Autodesk Inventor part; units mm, degrees
ref_plane "YZ Plane" through (0, 0, 0) normal (1, 0, 0) x (0, 1, 0)
ref_plane "XZ Plane" through (0, 0, 0) normal (0, 1, 0) x (-1, 0, 0)
ref_plane "XY Plane" through (0, 0, 0) normal (0, 0, 1) x (1, 0, 0)
sketch "Skizze2" plane through (0, 0, 0) normal (1, 0, 0) x (0, 1, 0)
  line L0 (1.25, 6) -> (-1.25, 6)
  line L1 (-1.25, 6) -> (-1.25, 0.25)
  line L2 (-1.25, 0.25) -> (-0.95, 0.25)
  line L3 (-0.95, 0.25) -> (-0.95, -0.25)
  line L4 (-0.95, -0.25) -> (-1.25, -0.25)
  line L5 (-1.25, -0.25) -> (-1.25, -6)
  line L6 (-1.25, -6) -> (1.25, -6)
  line L7 (1.25, -6) -> (1.25, -0.25)
  line L8 (1.25, -0.25) -> (0.95, -0.25)
  line L9 (0.95, -0.25) -> (0.95, 0.25)
  line L10 (0.95, 0.25) -> (1.25, 0.25)
  line L11 (1.25, 0.25) -> (1.25, 6)
  line L12 (0.25, 6) -> (0.25, -6) construction
  line L13 (-0.25, -6) -> (-0.25, 6) construction
  point P0 (0, 0)
  point P1 (0.95, 0)
  dimension "d0" = 0.5
  dimension "d1" = 1
  dimension "d2" = 1
  dimension "d3" = 0.5
  dimension "d4" = 0.25
  dimension "d5" = 0.3
  dimension "d6" = 0.3
  dimension "d7" = 6
  dimension "d8" = 6
extrude "Extrusion1" add sketch "Skizze2" along normal mid plane 12
sketch "Skizze3" plane through (-6, -1.25, -6) normal (0, 0, -1) x (-1, 0, 0)
  line L0 (-11, 1.5) -> (-1, 1.5)
  line L1 (-1, 1.5) -> (-1, 1)
  line L2 (-1, 1) -> (-11, 1)
  line L3 (-11, 1) -> (-11, 1.5)
  line L4 (0, 2.5) -> (-12, 2.5)
  line L5 (0, 2.5) -> (0, 0)
  point P0 (-6, 1.25)
  point P1 (-6, 1.5)
  point P2 (-6, 2.5)
  point P3 (-1, 1.25)
  point P4 (0, 1.25)
  dimension "d11" = 10
  dimension "d12" = 0.5
extrude "Extrusion2" cut sketch "Skizze3" against normal blind 12
sketch "Skizze4" plane through (-5, -0.25, -6) normal (0, 1, 0) x (1, 0, 0)
  line L0 (-1, -12) -> (11, -12)
  line L1 (-1, 0) -> (11, 0)
  line L2 (4.3, 0) -> (5.7, 0)
  line L3 (5.7, 0) -> (5.7, -12)
  line L4 (5.7, -12) -> (4.3, -12)
  line L5 (4.3, -12) -> (4.3, 0)
  line L6 (3.3, -12) -> (1.9, -12)
  line L7 (1.9, -12) -> (1.9, 0)
  line L8 (1.9, 0) -> (3.3, 0)
  line L9 (3.3, 0) -> (3.3, -12)
  line L10 (6.7, 0) -> (8.1, 0)
  line L11 (8.1, 0) -> (8.1, -12)
  line L12 (8.1, -12) -> (6.7, -12)
  line L13 (6.7, -12) -> (6.7, 0)
  point P0 (5, -6)
  point P1 (5, -12)
  point P2 (5, -12)
  dimension "d15" = 1.4
  dimension "d16" = 1
  dimension "d17" = 1
split_face "Trennen1"
split_face "Trennen2"
split_face "Trennen3"
equation "\"d2\" = d1"
equation "\"d6\" = d5"
equation "\"d17\" = d16"
properties part number "3_Pin_LED_Verbinder" material "PA 6.6"
The listing builds one solid part. Answer for the finished solid, in the listing's coordinates (mm). A direction names the side the tool comes from. Give positions to 0.01 mm unless a question says otherwise; leave off trailing zeros. Write each loop counter-clockwise with the first axis right and the second up, starting at its lowest first coordinate (ties: lowest second). Pieces come first, ordered by that corner, then holes. Notation, with made-up numbers: (74.5, 24.5) -> (98.5, 24.5) arc R26 ccw to (98.5, 55.5) -> close; hole circle Ø7 at (-7.75, -9.5). An arc over 180 degrees is marked (long way). One line per question, with ' | ' between items. Start each with the question number.
1. Find the intervals of material crossed by probe 1 along Y at (x, z) = (-3.5, -4); probe 2 along Z at (x, y) = (2, 1.1); probe 3 along X at (y, z) = (-0.05, 1.5), in increasing order.
2. Section B-B (x = 0.25) is taken. Determine the outline of the cut face in (y, z), plus the area to 3 significant figures.
3. For faces 1 (the flat face through (0, 1.25, 3)), 2 (the flat face through (0, -0.25, 0)), determine the directions among +Z, -Z, +X, -X, +Y, -Y from which every point of the face is accessible in a straight line to the end or side of a thin tool.
4. Section A-A (z = 0) is taken. Determine the outline of the cut face in (x, y), plus the area to 3 significant figures.
5. For a pull along Y with two mould halves and no side action, classify faces 3 (the flat face through (0, 0.25, 0)), 4 (the flat face through (0, -1, -6)), 5 (the flat face through (0, -1.25, -3)) as pulls with the +Y half, pulls with the -Y half, needs draft (parallel to the pull), parting line crosses it, or undercut.
Response values:
1) probe 1: -1.25 to -0.25, 0.25 to 1.25 | probe 2: -6 to -0.25, 0.25 to 6 | probe 3: -6 to -5, 5 to 6
2) outline: (-1.25, -6) -> (-0.25, -6) -> (-0.25, 6) -> (-1.25, 6) -> (-1.25, 0.25) -> (-0.95, 0.25) -> (-0.95, -0.25) -> (-1.25, -0.25) -> close; (0.25, -6) -> (1.25, -6) -> (1.25, -0.25) -> (0.95, -0.25) -> (0.95, 0.25) -> (1.25, 0.25) -> (1.25, 6) -> (0.25, 6) -> close | area: 23.7 mm2
3) face 1: +Z, -Z, +X, -X, +Y | face 2: +Z, -Z
4) outline: (-6, -0.95) -> (6, -0.95) -> (6, 0.95) -> (-6, 0.95) -> close; hole (-5, -0.25) -> (5, -0.25) -> (5, 0.25) -> (-5, 0.25) -> close | area: 17.8 mm2
5) face 3: undercut | face 4: needs draft | face 5: pulls with the -Y half
